```python
from build123d import *
from build123d.topology import SkipClean

# Parameters (mm, degrees)
SKETCH5_R           = 3.96875
EXTRUDE2_DEPTH      = 3
EXTRUDE2_DEPTH_BACK = 36.52
CHAMFER1_SIZE       = 1


with BuildPart() as part:
    # Sketch3 → Revolve2 (revolve)
    with BuildSketch(Plane(origin=(0, 0, 0), x_dir=(0, 0, -1), z_dir=(1, 0, 0))):
        with BuildLine():
            Line((-3.96875, 10.379628109), (-3.96875, 0))
            Line((-3.96875, 0), (3.96875, 0))
            Line((3.96875, 0), (3.96875, 10.379628109))
            ThreePointArc((3.96875, 10.379628109), (0, 11.1125), (-3.96875, 10.379628109))
        make_face()
    revolve(axis=Axis((0, 0, 8.146649187), (0, 0, -1)))

    # Sketch2 → Cut-Revolve2 (revolve, cut)
    with BuildSketch(Plane(origin=(0, 0, 0), x_dir=(0, 0, -1), z_dir=(1, 0, 0))):
        with BuildLine():
            Line((0, 7.5311), (0, -7.5311))
            ThreePointArc((0, -7.5311), (7.5311, 0), (0, 7.5311))
        make_face()
    revolve(axis=Axis((0, 15.474361319, 0), (0, -1, 0)), mode=Mode.SUBTRACT)

    # Sketch5 → Extrude2 (add, two sides)
    with SkipClean():  # the faces are left unmerged after this step: merging them gives an invalid solid
        with BuildSketch(Plane(origin=(0, -11.1125, 0), x_dir=(-1, 0, 0), z_dir=(0, 1, 0))) as extrude2_sk:
            with Locations(Location((0, 0, 0), (0, 0, 90))):
                Circle(SKETCH5_R)
        extrude(amount=EXTRUDE2_DEPTH)
        extrude(extrude2_sk.sketch, amount=-EXTRUDE2_DEPTH_BACK)

    # Chamfer1
    chamfer1_edges = [part.edges().sort_by_distance(p)[0] for p in [
        (0, -47.6325, -3.96875),
    ]]
    chamfer(chamfer1_edges, length=CHAMFER1_SIZE)


solid = part.part
```
Input: part model. Units: mm. Frame: model coordinates. Round coordinates to 2 decimals unless told otherwise and drop trailing zeros. Write each loop counter-clockwise with the first axis right and the second up, starting at its lowest first coordinate (ties: lowest second). Pieces come first, ordered by that corner, then holes. Notation, with made-up numbers: (-40, 55.5) - (6, 55.5) arc R27 ccw to (6, 91.5) - close; hole circle Ø8 at (65, 48). An arc over 180 degrees is marked (long way). Write item = value, one per line.
(1) Material intervals for probe 1 along X at (y, z) = (-5.5, -2.25); probe 2 along Y at (x, z) = (3.5, -3.25); probe 3 along Y at (x, z) = (1, 1.75), sorted ascending.
Geometry check:
probe_1 = -9.39 to -4.63, 4.63 to 9.39
probe_2 = -10.03 to -5.82, 5.82 to 10.03
probe_3 = -47.63 to -7.26, 7.26 to 10.93
(2) Section query B-B on z = 0. Output: boundary loops of the cut face in (x, y) (1 decimal), then the cut area to 3 significant figures.
Geometry check:
outline = (-4, -46.6) - (-3, -47.6) - (3, -47.6) - (4, -46.6) - (4, -10.4) arc R11.1 ccw (long way) to (-4, -10.4) - close; hole circle Ø15.1 at (0, 0)
area = 501 mm^2
(3) Section query D-D on y = -19. Output: boundary loops of the cut face in (x, z), then the cut area to 3 significant figures.
Geometry check:
outline = circle Ø7.94 at (0, 0)
area = 49.5 mm^2
(4) Contact query for flat-ended pins moving along their axis: pin 1 Ø1.5 at (x, y) = (4, -22) entering from -Z; pin 2 Ø3 at (x, y) = (-4.5, 0.5) entering from -Z; pin 3 Ø1.5 at (x, z) = (7.5, -2.5) entering from -Y; pin 4 Ø1 at (y, z) = (-1, -0.5) entering from +X. Output: stop coordinate, or through.
Geometry check:
pin_1 = -2.28
pin_2 = through
pin_3 = -8.5
pin_4 = 11.1
(5) Section query C-C on x = 4.5. Output: boundary loops of the cut face in (y, z), then the cut area to 3 significant figures.
Geometry check:
outline = (-9.35, -3.97) - (-4.55, -3.97) arc R6.04 cw to (-4.55, 3.97) - (-9.35, 3.97) arc R10.16 ccw to start; (4.55, -3.97) - (9.35, -3.97) arc R10.16 ccw to (9.35, 3.97) - (4.55, 3.97) arc R6.04 cw to start
area = 68.7 mm^2
(6) Section query A-A on y = 2. Output: boundary loops of the cut face in (x, z), then the cut area to 3 significant figures.
Geometry check:
outline = (-10.19, -3.97) - (-6.08, -3.97) arc R7.26 cw to (-6.08, 3.97) - (-10.19, 3.97) arc R10.93 ccw to start; (6.08, -3.97) - (10.19, -3.97) arc R10.93 ccw to (10.19, 3.97) - (6.08, 3.97) arc R7.26 cw to start
area = 60.4 mm^2
